from build123d import *

# Parameters (mm, degrees)
CROQUIS1_W                               = 300
CROQUIS1_H                               = 300
SALIENTE_EXTRUIR1_DEPTH                  = 15
CROQUIS2_W                               = 98
CROQUIS2_H                               = 98
SALIENTE_EXTRUIR2_DEPTH                  = 150
CROQUIS3_W                               = 40
CROQUIS3_H                               = 60
CROQUIS3_W_2                             = 20
CROQUIS3_H_2                             = 40
SALIENTE_EXTRUIR3_DEPTH                  = 30
CROQUIS4_W                               = 182
CROQUIS4_H                               = 80
CROQUIS4_W_2                             = 162
CROQUIS4_H_2                             = 60
SALIENTE_EXTRUIR4_DEPTH                  = 50
TALADRO_DE_MARGEN_PARA_M3_51_D           = 3.9
TALADRO_DE_MARGEN_PARA_M3_51_DEPTH       = 15
TALADRO_DE_MARGEN_PARA_M3_51_CSINK_D     = 3.95
TALADRO_DE_MARGEN_PARA_M3_51_CSINK_ANGLE = 90
TALADRO_DE_MARGEN_PARA_M3_51_TIP         = 1.171678207
CROQUIS7_W                               = 5
CROQUIS7_H                               = 7.608570781
CORTAR_EXTRUIR1_DEPTH                    = 10
CROQUIS8_W                               = 30
CROQUIS8_H                               = 15
CORTAR_EXTRUIR2_DEPTH                    = 10
CROQUIS9_R                               = 2
CORTAR_EXTRUIR3_DEPTH                    = 20


with BuildPart() as part:
    # Croquis1 → Saliente-Extruir1 (new body)
    with BuildSketch(Plane(origin=(0, 0, 0), x_dir=(1, 0, 0), z_dir=(0, 1, 0))):
        Rectangle(CROQUIS1_W, CROQUIS1_H)
    extrude(amount=SALIENTE_EXTRUIR1_DEPTH)

    # Croquis2 → Saliente-Extruir2 (add)
    with BuildSketch(Plane(origin=(0, 15, 0), x_dir=(1, 0, 0), z_dir=(0, 1, 0))):
        Polygon((-150, -140), (-150, -150), (-32, -150), (-32, -55), (-32, -32), (-150, -32), (-150, -55), align=None)
        with Locations((-91, -91)):
            Rectangle(CROQUIS2_W, CROQUIS2_H, mode=Mode.SUBTRACT)
    extrude(amount=SALIENTE_EXTRUIR2_DEPTH)

    # Croquis3 → Saliente-Extruir3 (add)
    with BuildSketch(Plane(origin=(0, 15, 0), x_dir=(1, 0, 0), z_dir=(0, 1, 0))):
        with Locations((0, 80)):
            Rectangle(CROQUIS3_W, CROQUIS3_H)
        with Locations((0, 80)):
            Rectangle(CROQUIS3_W_2, CROQUIS3_H_2, mode=Mode.SUBTRACT)
    extrude(amount=SALIENTE_EXTRUIR3_DEPTH)

    # Croquis4 → Saliente-Extruir4 (add)
    with BuildSketch(Plane(origin=(0, 15, 0), x_dir=(1, 0, 0), z_dir=(0, 1, 0))):
        with Locations((59, -110)):
            Rectangle(CROQUIS4_W, CROQUIS4_H)
        with Locations((59, -110)):
            Rectangle(CROQUIS4_W_2, CROQUIS4_H_2, mode=Mode.SUBTRACT)
    extrude(amount=SALIENTE_EXTRUIR4_DEPTH)

    # Taladro de margen para M3.51
    with Locations(Plane(origin=(0, 45, 0), x_dir=(1, 0, 0), z_dir=(0, 1, 0))):
        with Locations((-5, 104.25), (5, 104.25), (-5, 55.75), (5, 55.75)):
            CounterSinkHole(TALADRO_DE_MARGEN_PARA_M3_51_D / 2, TALADRO_DE_MARGEN_PARA_M3_51_CSINK_D / 2, depth=TALADRO_DE_MARGEN_PARA_M3_51_DEPTH, counter_sink_angle=TALADRO_DE_MARGEN_PARA_M3_51_CSINK_ANGLE)
            with Locations((0, 0, -(TALADRO_DE_MARGEN_PARA_M3_51_DEPTH + TALADRO_DE_MARGEN_PARA_M3_51_TIP / 2))):  # 118° drill point
                Cone(0, TALADRO_DE_MARGEN_PARA_M3_51_D / 2, TALADRO_DE_MARGEN_PARA_M3_51_TIP, mode=Mode.SUBTRACT)

    # Croquis7 → Cortar-Extruir1 (cut)
    with BuildSketch(Plane.XY.offset(-50)):
        with Locations((0, 18.373101355)):
            Rectangle(CROQUIS7_W, CROQUIS7_H)
    extrude(amount=-CORTAR_EXTRUIR1_DEPTH, mode=Mode.SUBTRACT)

    # Croquis8 → Cortar-Extruir2 (cut)
    with BuildSketch(Plane.XY.offset(80)):
        with Locations((18.908102742, 22.5)):
            Rectangle(CROQUIS8_W, CROQUIS8_H)
    extrude(amount=-CORTAR_EXTRUIR2_DEPTH, mode=Mode.SUBTRACT)

    # Croquis9 → Cortar-Extruir3 (cut)
    with BuildSketch(Plane(origin=(0, 15, 0), x_dir=(1, 0, 0), z_dir=(0, 1, 0))):
        with Locations((-140, 80)):
            Circle(CROQUIS9_R)
    extrude(amount=-CORTAR_EXTRUIR3_DEPTH, mode=Mode.SUBTRACT)


solid = part.part
Part model, mm, in its own coordinate system. A direction names the side the tool comes from. Coordinates: 2 decimals unless noted, no trailing zeros. Write each loop counter-clockwise with the first axis right and the second up, starting at its lowest first coordinate (ties: lowest second). Pieces come first, ordered by that corner, then holes. Notation, with made-up numbers: (13, 23) - (49, 23) arc R5 cw to (49, 30) - close; hole circle Ø7 at (-24.75, -19). An arc over 180 degrees is marked (long way). Put each result on its own line as item: value.
1. Band-saw the part on C-C (x = 95). Write the cut outline in (y, z), then the cut area to 3 significant figures.
Final values:
outline: (0, -150) - (15, -150) - (15, 70) - (65, 70) - (65, 80) - (15, 80) - (15, 140) - (65, 140) - (65, 150) - (0, 150) - close
area: 5,500 mm²
2. 3-axis set-ups, long thin cutter, end or side, ignore diameter. For faces 4 (the flat face through (2.5, 18, -55)), 5 (the flat face through (45, 65, 142)), 6 (the flat face through (0, 15, -80)): which of +Z, -Z, +X, -X, +Y, -Y reach the whole face in a straight line?
Final values:
face 4: none
face 5: +Z, -Z, +X, +Y
face 6: +Y
3. Two-plate mould, pull along Z, no slides. Class faces 1 (the flat face through (-2, 7, -150)), 2 (the flat face through (58, 40, 140)), 3 (the flat face through (-20, 30, -80)): +Z half, -Z half, draft (parallel to the pull), parting line (faces both ways), or undercut.
Final values:
face 1: -Z half
face 2: undercut
face 3: draft
4. Flat gauge pins, fed straight in: pin 1 Ø24 at (y, z) = (28.5, -65.5) entering from +X; pin 2 Ø12 at (y, z) = (51.5, 58.5) entering from +X; pin 3 Ø5 at (x, z) = (37, -36.5) entering from +Y. Where does each tip first touch, or does it go through?
Final values:
pin 1: stops at x = 20
pin 2: stops at x = -32
pin 3: stops at y = 15
5. Band-saw the part on A-A (x = 29). Write the cut outline in (y, z), then the cut area to 3 significant figures.
Final values:
outline: (0, -150) - (15, -150) - (15, 140) - (65, 140) - (65, 150) - (0, 150) - close; (30, 70) - (65, 70) - (65, 80) - (30, 80) - close
area: 5,350 mm²
6. Band-saw the part on B-B (y = 61). Write the cut outline in (x, z), then the cut area to 3 significant figures.
Final values:
outline: (-150, 32) - (-32, 32) - (-32, 70) - (150, 70) - (150, 150) - (-150, 150) - close; hole (-140, 42) - (-42, 42) - (-42, 140) - (-140, 140) - close; hole (-22, 80) - (140, 80) - (140, 140) - (-22, 140) - close
area: 9,160 mm²
7. Band-saw the part on D-D (y = 144). Write the cut outline in (x, z), then the cut area to 3 significant figures.
Final values:
outline: (-150, 32) - (-32, 32) - (-32, 150) - (-150, 150) - close; hole (-140, 42) - (-42, 42) - (-42, 140) - (-140, 140) - close
area: 4,320 mm²
8. Probe line 1 along Z through (x, y) = (-76.5, 103); line 2 along X through (y, z) = (89, 102); line 3 along X through (y, z) = (33, -55.75). List the from-to ranges inside material, lowest first. Write a range as [from, to].
Final values:
line 1: z = [32, 42], [140, 150]
line 2: x = [-150, -140], [-42, -32]
line 3: x = [-20, -6.95], [-3.05, 3.05], [6.95, 20]
